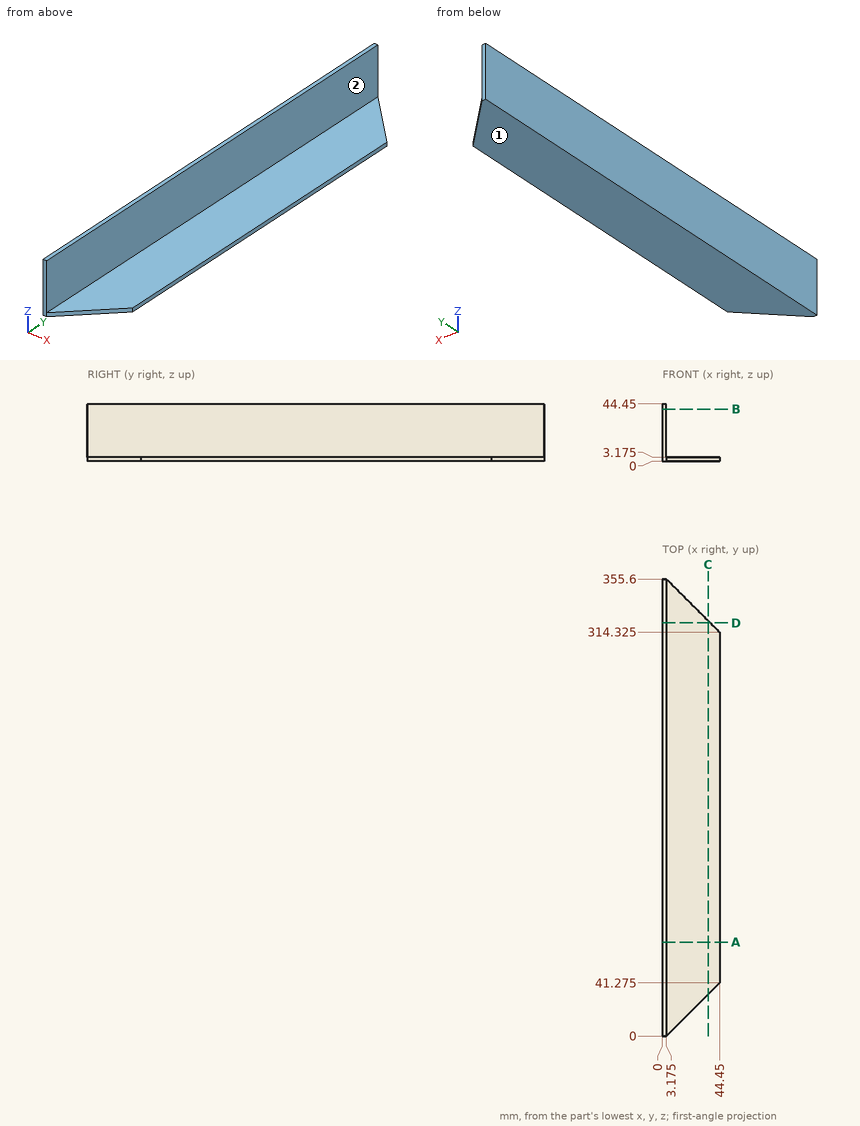
Drawing for the job (mm, zero at the part's lowest x, y, z). A direction names the side the tool comes from. Round coordinates to 2 decimals unless told otherwise and drop trailing zeros. Loops run counter-clockwise (first coordinate to the right, second up) from the corner with the lowest first, then second, coordinate; pieces in that order, holes last. Notation, with made-up numbers: (77, -21.75) -> (91, -21.75) arc R6 cw to (91, -10.75) -> close; hole circle Ø10 at (38.25, 1). An arc over 180 degrees is marked (long way). Answer in a Markdown table with one row per item.
Item 1: Saw through at C-C (x = 35.5). Write the cut outline in (y, z) (3 decimals).
Answers below:
| item | result |
|---|---|
| outline | (32.325, 0) -> (323.275, 0) -> (323.275, 3.175) -> (32.325, 3.175) -> close |
Item 2: Pin check, flat tips, straight feed: pin 1 (2 mm diameter, centred on x = 33.5, y = 182, fed in from +Z) (3 decimals); pin 2 (1 mm diameter, centred on y = 286.5, z = 27.5, fed in from +X) (3 decimals). Stop position of each tip, or through.
Answers below:
| item | result |
|---|---|
| pin 1 | stops at z = 3.175 |
| pin 2 | stops at x = 3.175 |
Item 3: Saw through at D-D (y = 321.5). Write the cut outline in (x, z) (3 decimals).
Answers below:
| item | result |
|---|---|
| outline | (0, 0) -> (37.275, 0) -> (37.275, 3.175) -> (3.175, 3.175) -> (3.175, 44.45) -> (0, 44.45) -> close |
Item 4: Saw through at A-A (y = 73). Write the cut outline in (x, z) (3 decimals).
Answers below:
| item | result |
|---|---|
| outline | (0, 0) -> (44.45, 0) -> (44.45, 3.175) -> (3.175, 3.175) -> (3.175, 44.45) -> (0, 44.45) -> close |
Item 5: Which spindle directions (+Z, -Z, +X, -X, +Y, -Y) get a long thin tool onto all of the face, cutting with end or side? Do the marked faces 1 and 2. Say none if no direction does.
Answers below:
| item | result |
|---|---|
| face 1 | -Z, +X, -X, +Y, -Y |
| face 2 | +Z, +X, +Y, -Y |
Item 6: Saw through at B-B (z = 40.5). Write the cut outline in (x, y) (3 decimals), and give its area (3 significant figures).
Answers below:
| item | result |
|---|---|
| outline | (0, 0) -> (3.175, 0) -> (3.175, 355.6) -> (0, 355.6) -> close |
| area | 1,130 mm² |
Item 7: Drill centre line: L1, parallel to X at y = 323, z = 4 (3 decimals). Where is it in solid material? Low to high. Write a range as [from, to].
Answers below:
| item | result |
|---|---|
| L1 | x = [0, 3.175] |
